```python
from build123d import *

# Parameters (mm, degrees)
SKETCH1_R          = 1.6
EXTRUDE2_DEPTH     = 3
CUT_EXTRUDE4_DEPTH = 3


with BuildPart() as part:
    # Sketch1 → Extrude2 (new body)
    with BuildSketch(Plane.XZ):
        Polygon((-21.510078765, -227.497048214), (2.632056859, -227.497048214), (53.489921235, -278.35491259), (53.489921235, -306.639183837), (2.632056859, -357.497048214), (-21.510078765, -357.497048214), (-21.510078765, -377.497048214), (32.129531542, -377.497048214), (55.092111961, -354.534467794), (176.887730509, -354.534467794), (199.850310928, -377.497048214), (253.489921235, -377.497048214), (253.489921235, -357.497048214), (229.347785611, -357.497048214), (178.489921235, -306.639183837), (178.489921235, -278.35491259), (229.347785611, -227.497048214), (253.489921235, -227.497048214), (253.489921235, -207.497048214), (199.850310928, -207.497048214), (176.887730509, -230.459628633), (55.092111961, -230.459628633), (32.129531542, -207.497048214), (-21.510078765, -207.497048214), align=None)
        with Locations((-11.510078765, -367.497048214)):
            Circle(SKETCH1_R, mode=Mode.SUBTRACT)
        with Locations((58.489921235, -292.497048214)):
            Circle(SKETCH1_R, mode=Mode.SUBTRACT)
        with Locations((243.489921235, -367.497048214)):
            Circle(SKETCH1_R, mode=Mode.SUBTRACT)
        with Locations((173.489921235, -292.497048214)):
            Circle(SKETCH1_R, mode=Mode.SUBTRACT)
        with Locations((-11.510078765, -217.497048214)):
            Circle(SKETCH1_R, mode=Mode.SUBTRACT)
        with Locations((243.489921235, -217.497048214)):
            Circle(SKETCH1_R, mode=Mode.SUBTRACT)
    extrude(amount=EXTRUDE2_DEPTH)

    # Sketch4 → Cut-Extrude4 (cut)
    with BuildSketch(Plane.XZ.offset(3)):
        with BuildLine():
            Line((121.389921235, -332.984350137), (121.389921235, -330.284350137))
            ThreePointArc((121.389921235, -330.284350137), (121.097028016, -329.577243356), (120.389921235, -329.284350137))
            Line((120.389921235, -329.284350137), (111.589921235, -329.284350137))
            ThreePointArc((111.589921235, -329.284350137), (110.882814454, -329.577243356), (110.589921235, -330.284350137))
            Line((110.589921235, -330.284350137), (110.589921235, -332.984350137))
            ThreePointArc((110.589921235, -332.984350137), (110.882814454, -333.691456918), (111.589921235, -333.984350137))
            Line((111.589921235, -333.984350137), (120.389921235, -333.984350137))
            ThreePointArc((120.389921235, -333.984350137), (121.097028016, -333.691456918), (121.389921235, -332.984350137))
        make_face()
        with BuildLine():
            ThreePointArc((142.489921235, -261.497048214), (140.989921235, -259.997048214), (139.489921235, -261.497048214))
            ThreePointArc((139.489921235, -261.497048214), (140.989921235, -262.997048214), (142.489921235, -261.497048214))
        make_face()
        with BuildLine():
            ThreePointArc((139.489921235, -323.497048214), (140.989921235, -324.997048214), (142.489921235, -323.497048214))
            ThreePointArc((142.489921235, -323.497048214), (140.989921235, -321.997048214), (139.489921235, -323.497048214))
        make_face()
        with BuildLine():
            ThreePointArc((92.489921235, -261.497048214), (90.989921235, -259.997048214), (89.489921235, -261.497048214))
            ThreePointArc((89.489921235, -261.497048214), (90.989921235, -262.997048214), (92.489921235, -261.497048214))
        make_face()
        with BuildLine():
            ThreePointArc((92.489921235, -323.497048214), (90.989921235, -321.997048214), (89.489921235, -323.497048214))
            ThreePointArc((89.489921235, -323.497048214), (90.989921235, -324.997048214), (92.489921235, -323.497048214))
        make_face()
    extrude(amount=-CUT_EXTRUDE4_DEPTH, mode=Mode.SUBTRACT)


solid = part.part
```
CAD build for the part. Positions are in the model's coordinates, mm. A direction names the side the tool comes from. Round coordinates to 2 decimals unless told otherwise and drop trailing zeros. Loops run counter-clockwise (first coordinate to the right, second up) from the corner with the lowest first, then second, coordinate; pieces in that order, holes last. Notation, with made-up numbers: (20, 32) - (77, 32) arc R24 ccw to (77, 51) - close; hole circle Ø6 at (17.25, 40). An arc over 180 degrees is marked (long way). Return JSON: item names as keys, results as strings. Group by question number.
Q1. Band-saw the part on D-D on z = -245. Give the cut face in (x, y) (3 decimals), plus the area to 3 significant figures.
Q2. Two-plate mould, pull along X, no slides. Class faces 1 (the face through (43.45, -1.479, -366.176)), 2 (the face through (188.208, -1.479, -365.855)), 3 (the face through (114, 0, -291)), 4 (the face through (203.563, -1.479, -253.282)): +X half, -X half, draft (parallel to the pull), parting line (faces both ways), or undercut.
Q3. Band-saw the part on C-C on x = 159. Give the cut face in (y, z), plus the area to 3 significant figures.
Q4. Flat gauge pins, fed straight in: pin 1 Ø1.3 at (y, z) = (-1, -331.5) entering from -X; pin 2 Ø1.5 at (x, y) = (117, -2) entering from -Z; pin 3 Ø1.3 at (y, z) = (-1.5, -331.5) entering from +X. Where does each tip first touch, or does it go through?
Q5. Drill centre lines: line 1 along X through (y, z) = (-1.6, -278.5); line 2 along Z through (x, y) = (62, -2); line 3 along Z through (x, y) = (207.5, -2.75). Where is each one in solid material? Low to high. Write a range as [from, to].
Q6. Band-saw the part on A-A on x = 8.5. Give the cut face in (y, z) (3 decimals), plus the area to 3 significant figures.
Q7. Tool access for faces 5 (the face through (204.27, -1.48, -332.42)), 6 (the face through (28.42, -1.48, -331.71)), 7 (the face through (43.77, -1.48, -219.14)): list every direction of +Z, -Z, +X, -X, +Y, -Y with a clear straight run to the whole face (end or side of a thin tool).
Q8. Band-saw the part on B-B on z = -222. Give the cut face in (x, y).
Solutions:
{
 "1": {"outline": "(20.135, -3) - (211.845, -3) - (211.845, 0) - (20.135, 0) - close", "area": "575 mm^2"},
 "2": {"face 1": "undercut", "face 2": "undercut", "face 3": "draft", "face 4": "+X half"},
 "3": {"outline": "(-3, -354.53) - (0, -354.53) - (0, -230.46) - (-3, -230.46) - close", "area": "372 mm^2"},
 "4": {"pin 1": "stops at x = 27.98", "pin 2": "stops at z = -354.53", "pin 3": "stops at x = 204"},
 "5": {"line 1": "x = [53.49, 178.49]", "line 2": "z = [-354.53, -230.46]", "line 3": "z = [-377.5, -335.65], [-249.34, -207.5]"},
 "6": {"outline": "(-3, -377.497) - (0, -377.497) - (0, -351.629) - (-3, -351.629) - close; (-3, -233.365) - (0, -233.365) - (0, -207.497) - (-3, -207.497) - close", "area": "155 mm^2"},
 "7": {"face 5": "+X, +Y, -Y", "face 6": "-X, +Y, -Y", "face 7": "+Z, +Y, -Y"},
 "8": {"outline": "(-21.51, -3) - (46.63, -3) - (46.63, 0) - (-21.51, 0) - close; (185.35, -3) - (253.49, -3) - (253.49, 0) - (185.35, 0) - close"}
}
